Model file for the job. Use its own axes, mm. Face numbers are marked on the shaded views. A direction names the side the tool comes from. Round coordinates to 2 decimals unless told otherwise and drop trailing zeros. Loops run counter-clockwise (first coordinate to the right, second up) from the corner with the lowest first, then second, coordinate; pieces in that order, holes last. Notation, with made-up numbers: M -27.75,60 L 8.25,60 A21 cw 8.25,78 Z; hole C 53,26.25 d7. An arc over 180 degrees is marked long. Use a Markdown table: item, result. Add a question column.
Item 1: Pin check, flat tips, straight feed: P1, Ø8, axis at x = 16, y = 8, coming from the +Z side; P2, Ø1.5, axis at x = -2.5, y = 4.5, coming from the +Z side; P3, Ø6, axis at x = 6.5, y = 11.5, coming from the +Z side. Stop position of each tip, or through.
Item 2: Wall check: L1, parallel to Z at x = -14.5, y = 1.5; L2, parallel to Z at x = 7, y = 2.5; L3, parallel to X at y = 11.5, z = 16. Give the ranges that are in metal, low to high. Write a range as from..to.
Item 3: Saw through at B-B on x = -14. Write the cut outline in (y, z).
Item 4: Tool access for the marked faces 1, 2 and 3: list every direction of +Z, -Z, +X, -X, +Y, -Y with a clear straight run to the whole face (end or side of a thin tool).
Item 5: Saw through at A-A on y = 15.25. Write the cut outline in (x, z).
```python
from build123d import *

# Parameters (mm, degrees)
CROQUIS1_W              = 40
CROQUIS1_H              = 20
SALIENTE_EXTRUIR1_DEPTH = 20
SALIENTE_EXTRUIR2_DEPTH = 20


with BuildPart() as part:
    # Croquis1 → Saliente-Extruir1 (new body)
    with BuildSketch(Plane(origin=(0, 0, 0), x_dir=(1, 0, 0), z_dir=(0, 1, 0))):
        Rectangle(CROQUIS1_W, CROQUIS1_H)
    extrude(amount=SALIENTE_EXTRUIR1_DEPTH)

    # Croquis2 → Saliente-Extruir2 (add)
    with BuildSketch(Plane(origin=(0, 20, 0), x_dir=(1, 0, 0), z_dir=(0, 1, 0))):
        with BuildLine():
            Line((-10, -10), (10, -10))
            ThreePointArc((10, -10), (0, -20), (-10, -10))
        make_face()
    extrude(amount=-SALIENTE_EXTRUIR2_DEPTH)


solid = part.part
```
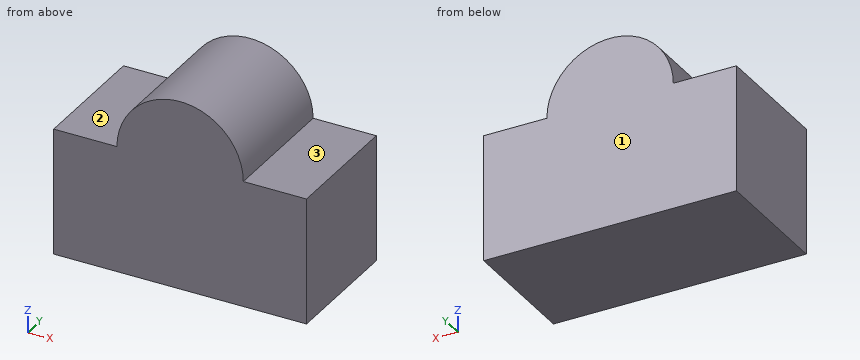
Entries:
| question | item | result |
|---|---|---|
| 1 | P1 | z = 10 |
| 1 | P2 | z = 19.85 |
| 1 | P3 | z = 19.37 |
| 2 | L1 | -10..10 |
| 2 | L2 | -10..17.14 |
| 2 | L3 | -8..8 |
| 3 | outline | M 0,-10 L 20,-10 L 20,10 L 0,10 Z |
| 4 | face 1 | +Z, -Z, +X, -X, +Y |
| 4 | face 2 | +Z, -X, +Y, -Y |
| 4 | face 3 | +Z, +X, +Y, -Y |
| 5 | outline | M -20,-10 L 20,-10 L 20,10 L 10,10 A10 ccw -10,10 L -20,10 Z |
